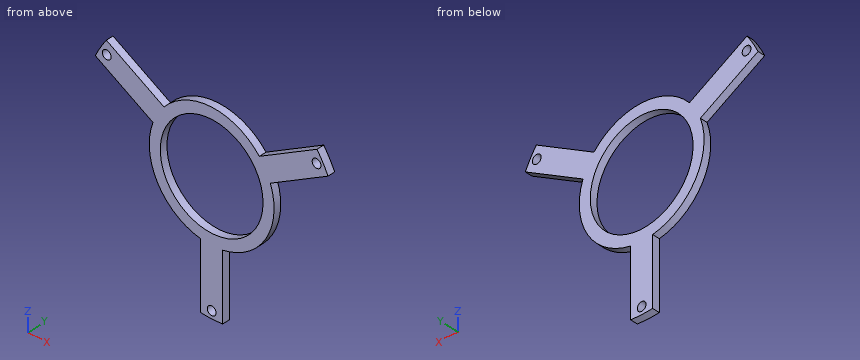
from build123d import *

# Parameters (mm, degrees)
SKETCH_1_R      = 70
SKETCH_1_R_2    = 6
EXTRUDE_1_DEPTH = 10


with BuildPart() as part:
    # 草图1 → 凸台-拉伸1 (new body)
    with BuildSketch(Plane(origin=(0, 0, 0), x_dir=(1, 0, 0), z_dir=(0, 1, 0))):
        with BuildLine():
            Line((143.496688705, -100.168359928), (64.956883731, -54.823382383))
            ThreePointArc((64.956883731, -54.823382383), (0, -85), (-64.956883731, -54.823382383))
            Line((-64.956883731, -54.823382383), (-143.496688705, -100.168359928))
            ThreePointArc((-143.496688705, -100.168359928), (-151.554445662, -87.5), (-158.496688705, -74.187597814))
            Line((-158.496688705, -74.187597814), (-79.956883731, -28.84262027))
            ThreePointArc((-79.956883731, -28.84262027), (-73.612159322, 42.5), (-15, 83.666002653))
            Line((-15, 83.666002653), (-15, 174.355957742))
            ThreePointArc((-15, 174.355957742), (0, 175), (15, 174.355957742))
            Line((15, 174.355957742), (15, 83.666002653))
            ThreePointArc((15, 83.666002653), (73.612159322, 42.5), (79.956883731, -28.84262027))
            Line((79.956883731, -28.84262027), (158.496688705, -74.187597814))
            ThreePointArc((158.496688705, -74.187597814), (151.554445662, -87.5), (143.496688705, -100.168359928))
        make_face()
        Circle(SKETCH_1_R, mode=Mode.SUBTRACT)
        with Locations((0, 165)):
            Circle(SKETCH_1_R_2, mode=Mode.SUBTRACT)
        with Locations((142.894191624, -82.5)):
            Circle(SKETCH_1_R_2, mode=Mode.SUBTRACT)
        with Locations((-142.894191624, -82.5)):
            Circle(SKETCH_1_R_2, mode=Mode.SUBTRACT)
    extrude(amount=EXTRUDE_1_DEPTH)


solid = part.part
Source: CAD feature listing. Evaluate the final solid. Frame: model axes, mm. Give positions to 0.01 mm unless a question says otherwise; leave off trailing zeros. Write each loop counter-clockwise with the first axis right and the second up, starting at its lowest first coordinate (ties: lowest second). Pieces come first, ordered by that corner, then holes. Notation, with made-up numbers: (54, 2) - (73, 2) arc R19 cw to (73, 34) - close; hole circle Ø1 at (32.5, 76). An arc over 180 degrees is marked (long way). Write item = value, one per line. Start each with the question number.
Q1. Cut plane B-B, the plane x = 0. Return loops of the section in (y, z), then the cut area to 3 significant figures.
Q2. Pin query (flat end, axial travel): pin 1 Ø9.5 at (x, z) = (0, -165) entering from +Y; pin 2 Ø6 at (x, y) = (-101, 6) entering from +Z; pin 3 Ø1.5 at (x, y) = (37.5, 7) entering from -Z; pin 4 Ø3 at (x, y) = (-93, 7) entering from +Z. Return the tip coordinate at first contact, or that it passes through.
Q3. Cut plane A-A, the plane z = 0. Return loops of the section in (x, y).
Q4. Cut plane C-C, the plane y = 5.5. Return loops of the section in (x, z), then the cut area to 3 significant figures.
Q5. Material intervals for probe 1 along Z at (x, y) = (-0.5, 5); probe 2 along X at (y, z) = (3, -165); probe 3 along Z at (x, y) = (2.5, 6), sorted ascending.
Q6. Cut plane D-D, the plane z = 60. Return loops of the section in (x, y), then the cut area to 3 significant figures.
Computed values:
q1.outline = (0, -175) - (10, -175) - (10, -171) - (0, -171) - close; (0, -159) - (10, -159) - (10, -70) - (0, -70) - close; (0, 70) - (10, 70) - (10, 85) - (0, 85) - close
q1.area = 1,080 mm²
q2.pin_1 = through
q2.pin_2 = 77.36
q2.pin_3 = -76.64
q2.pin_4 = 71.88
q3.outline = (-85, 0) - (-70, 0) - (-70, 10) - (-85, 10) - close; (70, 0) - (85, 0) - (85, 10) - (70, 10) - close
q4.outline = (-158.5, 74.19) - (-79.96, 28.84) arc R85 ccw to (-15, -83.67) - (-15, -174.36) arc R175 ccw to (15, -174.36) - (15, -83.67) arc R85 ccw to (79.96, 28.84) - (158.5, 74.19) arc R175 ccw to (143.5, 100.17) - (64.96, 54.82) arc R85 ccw to (-64.96, 54.82) - (-143.5, 100.17) arc R175 ccw to start; hole circle Ø12 at (-142.89, 82.5); hole circle Ø140 at (0, 0); hole circle Ø12 at (0, -165); hole circle Ø12 at (142.89, 82.5)
q4.area = 15,100 mm²
q5.probe_1 = -175 to -170.98, -159.02 to -70, 70 to 85
q5.probe_2 = -15 to -6, 6 to 15
q5.probe_3 = -174.98 to -170.45, -159.55 to -69.96, 69.96 to 84.96
q6.outline = (-133.92, 0) - (-73.92, 0) - (-73.92, 10) - (-133.92, 10) - close; (-60.21, 0) - (-36.06, 0) - (-36.06, 10) - (-60.21, 10) - close; (36.06, 0) - (60.21, 0) - (60.21, 10) - (36.06, 10) - close; (73.92, 0) - (133.92, 0) - (133.92, 10) - (73.92, 10) - close
q6.area = 1,680 mm²
